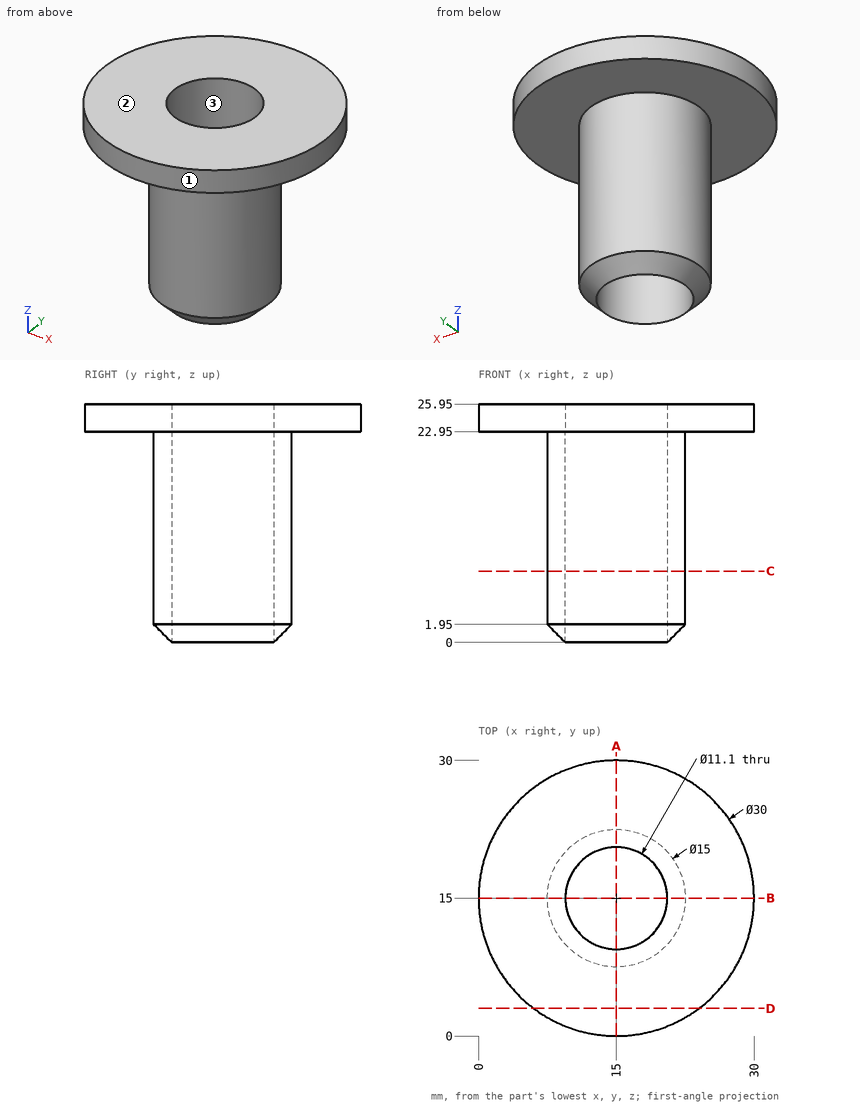
Could you check a few things on this drawing? It's one solid part, dimensions in mm from its lowest x, y, z. Round coordinates to 2 decimals unless told otherwise and drop trailing zeros. Loops run counter-clockwise (first coordinate to the right, second up) from the corner with the lowest first, then second, coordinate; pieces in that order, holes last.
Q1. Please list where these lines run through material, in increasing order: L1, parallel to Y at x = 15, z = 13; L2, parallel to Z at x = 5.25, y = 23.5; L3, parallel to X at y = 17, z = 15.
Q2. Thinking about a two-plate mould opening in Y: for the marked faces 1, 2 and 3, which applies, pulls with the +Y half, pulls with the -Y half, needs draft (parallel to the pull), parting line crosses it, or undercut?
Q3. For P1, Ø1, axis at x = 20, y = 5, coming from the -Z side; P2, Ø2, axis at x = 5.5, z = 9, coming from the -Y side; P3, Ø5, axis at y = 14.5, z = 2.5, coming from the -X side; P4, Ø15, axis at x = 7.5, y = 18, coming from the -Z side, each with a flat end and sliding along its axis, tell me the tip position at first contact or that it passes through.
Q4. I want a section at C-C (z = 7.75). Write out the boundary of the cut face in (x, y), and give its area (3 significant figures).
Q5. I want a section at D-D (y = 3). Write out the boundary of the cut face in (x, z).
Q6. I want a section at A-A (x = 15). Write out the boundary of the cut face in (y, z), and give its area (3 significant figures).
Answer below:
1. L1: y = 7.5 to 9.45, 20.55 to 22.5
1. L2: z = 22.95 to 25.95
1. L3: x = 7.77 to 9.82, 20.18 to 22.23
2. face 1: parting line crosses it
2. face 2: needs draft
2. face 3: undercut
3. P1: stops at z = 22.95
3. P2: passes through
3. P3: stops at x = 7.5
3. P4: stops at z = 0
4. outline: circle Ø15 at (15, 15); hole circle Ø11.1 at (15, 15)
4. area: 79.9 mm2
5. outline: (6, 22.95) - (24, 22.95) - (24, 25.95) - (6, 25.95) - close
6. outline: (0, 22.95) - (7.5, 22.95) - (7.5, 1.95) - (9.45, 0) - (9.45, 25.95) - (0, 25.95) - close; (20.55, 0) - (22.5, 1.95) - (22.5, 22.95) - (30, 22.95) - (30, 25.95) - (20.55, 25.95) - close
6. area: 142 mm2
